Geometry check sheet. Reference: the model listing, model coordinates, mm. Face numbers are marked on the shaded views. A direction names the side the tool comes from. Give positions to 0.01 mm unless a question says otherwise; leave off trailing zeros. Loops run counter-clockwise (first coordinate to the right, second up) from the corner with the lowest first, then second, coordinate; pieces in that order, holes last. Notation, with made-up numbers: (-15.75, -7.75) -> (4.25, -7.75) arc R10 cw to (4.25, 8.25) -> close; hole circle Ø4 at (-40, 57.25). An arc over 180 degrees is marked (long way). Write item = value, one per line.
```python
from build123d import *

# Parameters (mm, degrees)
BOSS_EXTRUDE1_DEPTH     = 7.62
SKETCH5_W               = 2.54
SKETCH5_H               = 12.7
CUT_EXTRUDE2_DEPTH      = 5.08
CUT_EXTRUDE3_DEPTH      = 34.408483952
CUT_EXTRUDE3_DEPTH_BACK = 34.408483952
SKETCH6_W               = 2.54
SKETCH6_H               = 1.058333333


with BuildPart() as part:
    # Sketch2 → Boss-Extrude1 (new body)
    with BuildSketch(Plane.XY):
        Polygon((0, 0), (-30.48, 0), (-15.24, 12.7), align=None)
    extrude(amount=BOSS_EXTRUDE1_DEPTH)

    # Sketch5 → Cut-Extrude2 (cut)
    with BuildSketch(Plane(origin=(0, 0, 0), x_dir=(-1, 0, 0), z_dir=(0, 0, -1))):
        with Locations((15.24, 6.35)):
            Rectangle(SKETCH5_W, SKETCH5_H)
    extrude(amount=-CUT_EXTRUDE2_DEPTH, mode=Mode.SUBTRACT)

    # Sketch6 → Cut-Extrude3 (cut, two sides: drawn at the far end of the back side and taken through both)
    with BuildSketch(Plane(origin=(0, 0, 5.08), x_dir=(-1, 0, 0), z_dir=(0, 0, -1)).offset(-CUT_EXTRUDE3_DEPTH_BACK)):
        with Locations((15.24, 12.170833334)):
            Rectangle(SKETCH6_W, SKETCH6_H)
    extrude(amount=CUT_EXTRUDE3_DEPTH + CUT_EXTRUDE3_DEPTH_BACK, mode=Mode.SUBTRACT)


solid = part.part
```
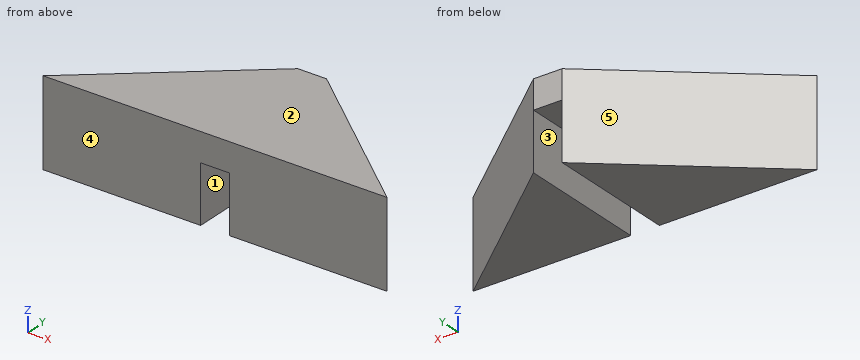
Item 1: Section check C-C, the plane x = -18. Record the cut outline in (y, z), plus the area to 3 significant figures.
Answer:
outline = (0, 0) -> (10.4, 0) -> (10.4, 7.62) -> (0, 7.62) -> close
area = 79.2 mm^2
Item 2: Thickness scan on L1, parallel to X at y = 6.5, z = 4; L2, parallel to X at y = 3.5, z = 1.75; L3, parallel to Z at x = -16, y = 10. Record the ranges inside material, lowest first. Write a range as [from, to].
Answer:
L1 = [-22.68, -16.51], [-13.97, -7.8]
L2 = [-26.28, -16.51], [-13.97, -4.2]
L3 = [5.08, 7.62]
Item 3: Draft check along X on the marked faces 3, 4 and 5. Enter one of: +X half, -X half, draft (parallel to the pull), parting line (faces both ways), or undercut.
Answer:
face_3 = undercut
face_4 = draft
face_5 = -X half
Item 4: Section check A-A, the plane z = 3.5. Record the cut outline in (x, y), plus the area to 3 significant figures.
Answer:
outline = (-30.48, 0) -> (-16.51, 0) -> (-16.51, 11.64) -> close; (-13.97, 0) -> (0, 0) -> (-13.97, 11.64) -> close
area = 163 mm^2
Item 5: Gauge pin test, flat ends, axial feed: pin 1 (3 mm diameter, centred on y = 6, z = 1, fed in from -X); pin 2 (2 mm diameter, centred on y = 2, z = 4.5, fed in from -X); pin 3 (1.5 mm diameter, centred on y = 8.5, z = 5.5, fed in from -X). Record the tip position at first contact, or that the pin passes through.
Answer:
pin_1 = -25.08
pin_2 = -29.28
pin_3 = -21.18
Item 6: Tool access check on the marked faces 1 and 2. Record the directions out of +Z, -Z, +X, -X, +Y, -Y that give a thin tool (end or side, any length) a straight path to the whole face; none if there is none.
Answer:
face_1 = -Z, +Y, -Y
face_2 = +Z, +X, -X, +Y, -Y
Item 7: Section check B-B, the plane y = 1.25. Record the cut outline in (x, z), plus the area to 3 significant figures.
Answer:
outline = (-28.98, 0) -> (-16.51, 0) -> (-16.51, 5.08) -> (-13.97, 5.08) -> (-13.97, 0) -> (-1.5, 0) -> (-1.5, 7.62) -> (-28.98, 7.62) -> close
area = 196 mm^2
Item 8: Section check D-D, the plane z = 6.25. Record the cut outline in (x, y), plus the area to 3 significant figures.
Answer:
outline = (-30.48, 0) -> (0, 0) -> (-13.97, 11.64) -> (-16.51, 11.64) -> close
area = 192 mm^2
